Can you work these out from the model? Positions are in its coordinate system, mm. Give positions to 0.01 mm unless a question says otherwise; leave off trailing zeros. Order: outer loops, then holes, each group sorted by start corner. A loop starts at its lowest first (then second) coordinate and runs counter-clockwise, first axis right, second up. Notation, with made-up numbers: (62, 57.25) - (110, 57.25) arc R4 cw to (110, 64.25) - close; hole circle Ø4 at (15, 42.25). An arc over 180 degrees is marked (long way). Return JSON: item names as keys, results as strings.
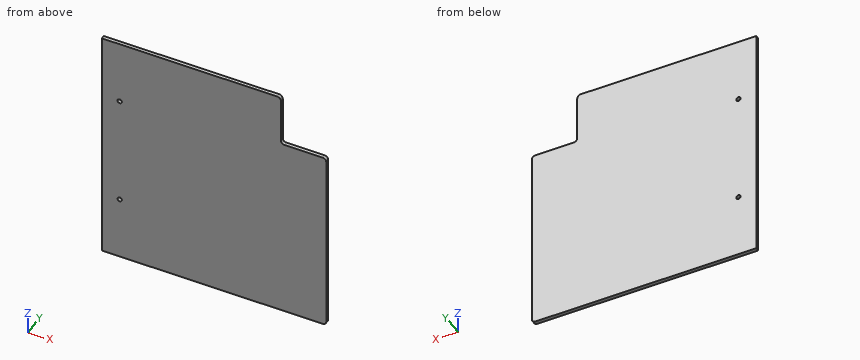
```python
from build123d import *

# Parameters (mm, degrees)
CROQUIS1_R              = 3
SALIENTE_EXTRUIR1_DEPTH = 5
REDONDEO1_R             = 5


with BuildPart() as part:
    # Croquis1 → Saliente-Extruir1 (new body)
    with BuildSketch(Plane(origin=(0, 0, 0), x_dir=(1, 0, 0), z_dir=(0, 1, 0))):
        Polygon((-117.776848249, -199.571984436), (-117.776848249, 134.928015564), (191.223151751, 134.928015564), (191.223151751, -127.071984436), (128.723151751, -127.071984436), (128.723151751, -199.571984436), align=None)
        with Locations(Location((-93.276848249, 44.928015564, 0), (0, 0, 270))):
            Circle(CROQUIS1_R, mode=Mode.SUBTRACT)
        with Locations(Location((-93.276848249, -109.571984436, 0), (0, 0, 270))):
            Circle(CROQUIS1_R, mode=Mode.SUBTRACT)
    extrude(amount=SALIENTE_EXTRUIR1_DEPTH)

    # Redondeo1
    redondeo1_edges = [part.edges().sort_by_distance(p)[0] for p in [
        (191.223151751, 2.5, 127.071984436),
        (128.723151751, 2.5, 127.071984436),
        (128.723151751, 2.5, 199.571984436),
        (191.223151751, 2.5, -134.928015564),
    ]]
    fillet(redondeo1_edges, radius=REDONDEO1_R)


solid = part.part
```
1. If I drill on L1, parallel to Z at x = 160.5, y = 0.8; L2, parallel to X at y = 2.9, z = 153; L3, parallel to Z at x = 131, y = 0.7, over which ranges is the centre line in solid material (lowest first)? Write a range as [from, to].
Checks:
{"L1": "[-134.93, 127.07]", "L2": "[-117.78, 128.72]", "L3": "[-134.93, 127.88]"}
2. Suppose I cut it at B-B (z = 152). List the corners of the cut face in (x, y) for me, plus the area to 3 significant figures.
Checks:
{"outline": "(-117.78, 0) - (128.72, 0) - (128.72, 5) - (-117.78, 5) - close", "area": "1,230 mm^2"}
3. Suppose I cut it at A-A (y = 3.35). List the corners of the cut face in (x, z) for me.
Checks:
{"outline": "(-117.78, -134.93) - (186.22, -134.93) arc R5 ccw to (191.22, -129.93) - (191.22, 122.07) arc R5 ccw to (186.22, 127.07) - (133.72, 127.07) arc R5 cw to (128.72, 132.07) - (128.72, 194.57) arc R5 ccw to (123.72, 199.57) - (-117.78, 199.57) - close; hole circle Ø6 at (-93.28, -44.93); hole circle Ø6 at (-93.28, 109.57)"}
4. For pin 1 Ø3.5 at (x, z) = (-93.28, 109.57) entering from -Y (1 decimal); pin 2 Ø1 at (x, y) = (135.5, 2) entering from +Z; pin 3 Ø6 at (x, z) = (-2, 37.5) entering from -Y; pin 4 Ø3 at (y, z) = (3, 151) entering from +X, each with a flat end and sliding along its axis, tell me the tip position at first contact or that it passes through.
Checks:
{"pin 1": "through", "pin 2": "z = 127.07", "pin 3": "y = 0", "pin 4": "x = 128.72"}
